Could you check a few things on this model? Use its own coordinates, in mm. A direction names the side the tool comes from. Round coordinates to 2 decimals unless told otherwise and drop trailing zeros. Order: outer loops, then holes, each group sorted by start corner. A loop starts at its lowest first (then second) coordinate and runs counter-clockwise, first axis right, second up. Notation, with made-up numbers: (41.25, -37.5) - (89.25, -37.5) arc R24 cw to (89.25, -18.5) - close; hole circle Ø5 at (56, 68). An arc over 180 degrees is marked (long way). Return JSON: item names as keys, results as strings. Group by question number.
from build123d import *

# Parameters (mm, degrees)
SKETCH1_R           = 0.95
SKETCH1_R_2         = 2.5
SKETCH1_R_3         = 1.449999999
SKETCH1_R_4         = 1.45
SKETCH1_W           = 6.2
SKETCH1_H           = 3.4
BOSS_EXTRUDE1_DEPTH = 5.85
FILLET1_R           = 4


with BuildPart() as part:
    # Sketch1 → Boss-Extrude1 (new body)
    with BuildSketch(Plane.XY):
        with BuildLine():
            Line((576.616706289, 434.650231372), (532.426650002, 446.716128422))
            ThreePointArc((532.426650002, 446.716128422), (529.426650002, 450.550186325), (532.426650002, 454.384244227))
            Line((532.426650002, 454.384244227), (576.616706289, 466.450141278))
            ThreePointArc((576.616706289, 466.450141278), (587.144059076, 475.326320371), (587.176754813, 489.096238418))
            Line((587.176754813, 489.096238418), (568.014947547, 530.703594601))
            ThreePointArc((568.014947547, 530.703594601), (569.023643468, 535.466212845), (573.889065048, 535.63256443))
            Line((573.889065048, 535.63256443), (611.536899087, 509.536826494))
            ThreePointArc((611.536899087, 509.536826494), (640.276650002, 500.550186325), (669.016400917, 509.536826494))
            Line((669.016400917, 509.536826494), (706.664234956, 535.63256443))
            ThreePointArc((706.664234956, 535.63256443), (711.529656536, 535.466212845), (712.538352458, 530.703594601))
            Line((712.538352458, 530.703594601), (693.376545192, 489.096238418))
            ThreePointArc((693.376545192, 489.096238418), (693.409240928, 475.326320371), (703.936593716, 466.450141278))
            Line((703.936593716, 466.450141278), (748.126650002, 454.384244227))
            ThreePointArc((748.126650002, 454.384244227), (751.126650002, 450.550186325), (748.126650002, 446.716128422))
            Line((748.126650002, 446.716128422), (703.936593716, 434.650231372))
            ThreePointArc((703.936593716, 434.650231372), (693.409240928, 425.774052279), (693.376545192, 412.004134232))
            Line((693.376545192, 412.004134232), (712.538352458, 370.396778049))
            ThreePointArc((712.538352458, 370.396778049), (711.529656536, 365.634159805), (706.664234956, 365.46780822))
            Line((706.664234956, 365.46780822), (683.276650002, 381.679000803))
            ThreePointArc((683.276650002, 381.679000803), (677.397639803, 388.334757147), (675.276650002, 396.958170375))
            Line((675.276650002, 396.958170375), (675.276650002, 489.550186325))
            Line((675.276650002, 489.550186325), (605.276650002, 489.550186325))
            Line((605.276650002, 489.550186325), (605.276650002, 396.958170375))
            ThreePointArc((605.276650002, 396.958170375), (603.155660202, 388.334757147), (597.276650002, 381.679000803))
            Line((597.276650002, 381.679000803), (573.889065048, 365.46780822))
            ThreePointArc((573.889065048, 365.46780822), (569.023643468, 365.634159805), (568.014947547, 370.396778049))
            Line((568.014947547, 370.396778049), (587.176754813, 412.004134232))
            ThreePointArc((587.176754813, 412.004134232), (587.144059076, 425.774052279), (576.616706289, 434.650231372))
        make_face()
        with Locations((533.376650002, 450.550186325)):
            Circle(SKETCH1_R, mode=Mode.SUBTRACT)
        with Locations((575.997889034, 527.154630637)):
            Circle(SKETCH1_R_2, mode=Mode.SUBTRACT)
        with Locations((547.176650002, 450.550186325)):
            Circle(SKETCH1_R, mode=Mode.SUBTRACT)
        with Locations((540.276650002, 450.550186325)):
            Circle(SKETCH1_R_2, mode=Mode.SUBTRACT)
        with Locations((590.276650002, 460.550186325)):
            Circle(SKETCH1_R_3, mode=Mode.SUBTRACT)
        with Locations((571.562654527, 532.440337294)):
            Circle(SKETCH1_R, mode=Mode.SUBTRACT)
        with Locations((580.43312354, 521.868923979)):
            Circle(SKETCH1_R, mode=Mode.SUBTRACT)
        with Locations(Location((682.276650002, 470.550186325, 0), (0, 0, 180))):
            Circle(SKETCH1_R_4, mode=Mode.SUBTRACT)
        with Locations((630.276650002, 494.550186325)):
            Circle(SKETCH1_R_4, mode=Mode.SUBTRACT)
        with Locations((620.276650002, 494.550186325)):
            Circle(SKETCH1_R_4, mode=Mode.SUBTRACT)
        with Locations((580.43312354, 379.231448671)):
            Circle(SKETCH1_R, mode=Mode.SUBTRACT)
        with Locations((575.997889034, 373.945742013)):
            Circle(SKETCH1_R_2, mode=Mode.SUBTRACT)
        with Locations((571.562654527, 368.660035356)):
            Circle(SKETCH1_R, mode=Mode.SUBTRACT)
        with Locations(Location((590.276650002, 430.550186325, 0), (0, 0, 180))):
            Circle(SKETCH1_R_3, mode=Mode.SUBTRACT)
        with Locations(Location((590.276650002, 440.550186325, 0), (0, 0, 180))):
            Circle(SKETCH1_R_3, mode=Mode.SUBTRACT)
        with Locations((590.276650002, 470.550186325)):
            Circle(SKETCH1_R_3, mode=Mode.SUBTRACT)
        with Locations(Location((682.276650002, 430.550186325, 0), (0, 0, 180))):
            Circle(SKETCH1_R_4, mode=Mode.SUBTRACT)
        with Locations(Location((708.990645478, 368.660035356, 0), (0, 0, 180))):
            Circle(SKETCH1_R, mode=Mode.SUBTRACT)
        with Locations(Location((704.555410971, 373.945742013, 0), (0, 0, 180))):
            Circle(SKETCH1_R_2, mode=Mode.SUBTRACT)
        with Locations(Location((700.120176464, 379.231448671, 0), (0, 0, 180))):
            Circle(SKETCH1_R, mode=Mode.SUBTRACT)
        with Locations(Location((660.276650002, 494.550186325, 0), (0, 0, 180))):
            Circle(SKETCH1_R_4, mode=Mode.SUBTRACT)
        with Locations(Location((650.276650002, 494.550186325, 0), (0, 0, 180))):
            Circle(SKETCH1_R_4, mode=Mode.SUBTRACT)
        with Locations(Location((700.120176464, 521.868923979, 0), (0, 0, 180))):
            Circle(SKETCH1_R, mode=Mode.SUBTRACT)
        with Locations(Location((708.990645478, 532.440337294, 0), (0, 0, 180))):
            Circle(SKETCH1_R, mode=Mode.SUBTRACT)
        with Locations(Location((690.276650002, 450.550186325, 0), (0, 0, 180))):
            Circle(SKETCH1_R_3, mode=Mode.SUBTRACT)
        with Locations(Location((740.276650002, 450.550186325, 0), (0, 0, 180))):
            Circle(SKETCH1_R_2, mode=Mode.SUBTRACT)
        with Locations(Location((733.376650002, 450.550186325, 0), (0, 0, 180))):
            Circle(SKETCH1_R, mode=Mode.SUBTRACT)
        with Locations(Location((704.555410971, 527.154630637, 0), (0, 0, 180))):
            Circle(SKETCH1_R_2, mode=Mode.SUBTRACT)
        with Locations(Location((747.176650002, 450.550186325, 0), (0, 0, 180))):
            Circle(SKETCH1_R, mode=Mode.SUBTRACT)
        with Locations(Location((690.276650002, 470.550186325, 0), (0, 0, 180))):
            Circle(SKETCH1_R_3, mode=Mode.SUBTRACT)
        with Locations((640.276650002, 494.550186325)):
            Circle(SKETCH1_R_4, mode=Mode.SUBTRACT)
        with Locations((690.276650002, 440.550186325)):
            Circle(SKETCH1_R_3, mode=Mode.SUBTRACT)
        with Locations((690.276650002, 430.550186325)):
            Circle(SKETCH1_R_3, mode=Mode.SUBTRACT)
        with Locations(Location((690.276650002, 460.550186325, 0), (0, 0, 180))):
            Circle(SKETCH1_R_3, mode=Mode.SUBTRACT)
        with Locations((590.276650002, 450.550186325)):
            Circle(SKETCH1_R_3, mode=Mode.SUBTRACT)
        with Locations((598.276650002, 430.550186325)):
            Circle(SKETCH1_R_4, mode=Mode.SUBTRACT)
        with Locations((598.276650002, 470.550186325)):
            Circle(SKETCH1_R_4, mode=Mode.SUBTRACT)
        with BuildLine():
            Line((549.378217697, 453.82975942), (576.389421361, 461.205047663))
            ThreePointArc((576.389421361, 461.205047663), (580.337323048, 460.434368256), (582.12067631, 456.828882764))
            Line((582.12067631, 456.828882764), (582.12067631, 444.271489885))
            ThreePointArc((582.12067631, 444.271489885), (580.337323048, 440.666004394), (576.389421361, 439.895324987))
            Line((576.389421361, 439.895324987), (549.378217697, 447.27061323))
            ThreePointArc((549.378217697, 447.27061323), (551.126650002, 450.550186325), (549.378217697, 453.82975942))
        make_face(mode=Mode.SUBTRACT)
        with BuildLine():
            Line((590.015887334, 402.739634304), (597.776650002, 402.739634304))
            ThreePointArc((597.776650002, 402.739634304), (599.544416955, 402.007401257), (600.276650002, 400.239634304))
            Line((600.276650002, 400.239634304), (600.276650002, 396.958170375))
            ThreePointArc((600.276650002, 396.958170375), (598.726100476, 390.65402441), (594.428250258, 385.788333948))
            Line((594.428250258, 385.788333948), (586.310038369, 380.161164806))
            ThreePointArc((586.310038369, 380.161164806), (584.257709818, 383.789413107), (580.328199648, 385.180523471))
            Line((580.328199648, 385.180523471), (587.745126051, 401.285408274))
            ThreePointArc((587.745126051, 401.285408274), (588.667635675, 402.34491753), (590.015887334, 402.739634304))
        make_face(mode=Mode.SUBTRACT)
        with Locations((598.276650002, 420.515790438)):
            Rectangle(SKETCH1_W, SKETCH1_H, mode=Mode.SUBTRACT)
        with BuildLine():
            Line((694.243261635, 380.161164806), (686.125049746, 385.788333948))
            ThreePointArc((686.125049746, 385.788333948), (681.827199528, 390.65402441), (680.276650002, 396.958170375))
            Line((680.276650002, 396.958170375), (680.276650002, 400.239634304))
            ThreePointArc((680.276650002, 400.239634304), (681.008883049, 402.007401257), (682.776650002, 402.739634304))
            Line((682.776650002, 402.739634304), (690.53741267, 402.739634304))
            ThreePointArc((690.53741267, 402.739634304), (691.88566433, 402.34491753), (692.808173953, 401.285408274))
            Line((692.808173953, 401.285408274), (700.225100356, 385.180523471))
            ThreePointArc((700.225100356, 385.180523471), (696.295590186, 383.789413107), (694.243261635, 380.161164806))
        make_face(mode=Mode.SUBTRACT)
        with BuildLine():
            Line((579.335965232, 518.07435633), (591.048633694, 492.641829961))
            ThreePointArc((591.048633694, 492.641829961), (594.150648115, 490.133983107), (598.026414137, 491.077501553))
            Line((598.026414137, 491.077501553), (607.701712221, 499.196040607))
            ThreePointArc((607.701712221, 499.196040607), (609.303916208, 502.849084775), (607.372828334, 506.339455663))
            Line((607.372828334, 506.339455663), (584.360562722, 522.29049423))
            ThreePointArc((584.360562722, 522.29049423), (582.972134599, 518.843048429), (579.335965232, 518.07435633))
        make_face(mode=Mode.SUBTRACT)
        with Locations((682.276650002, 480.550186325)):
            Rectangle(SKETCH1_W, SKETCH1_H, mode=Mode.SUBTRACT)
        with BuildLine():
            Line((672.851587783, 499.196040607), (682.526885868, 491.077501553))
            ThreePointArc((682.526885868, 491.077501553), (686.402651889, 490.133983107), (689.50466631, 492.641829961))
            Line((689.50466631, 492.641829961), (701.217334773, 518.07435633))
            ThreePointArc((701.217334773, 518.07435633), (697.581165406, 518.843048429), (696.192737283, 522.29049423))
            Line((696.192737283, 522.29049423), (673.18047167, 506.339455663))
            ThreePointArc((673.18047167, 506.339455663), (671.249383797, 502.849084775), (672.851587783, 499.196040607))
        make_face(mode=Mode.SUBTRACT)
        with BuildLine():
            Line((698.432623695, 456.828882764), (698.432623695, 444.271489885))
            ThreePointArc((698.432623695, 444.271489885), (700.215976956, 440.666004394), (704.163878644, 439.895324987))
            Line((704.163878644, 439.895324987), (731.175082307, 447.27061323))
            ThreePointArc((731.175082307, 447.27061323), (729.426650002, 450.550186325), (731.175082307, 453.82975942))
            Line((731.175082307, 453.82975942), (704.163878644, 461.205047663))
            ThreePointArc((704.163878644, 461.205047663), (700.215976956, 460.434368256), (698.432623695, 456.828882764))
        make_face(mode=Mode.SUBTRACT)
        with Locations((682.276650002, 420.515790438)):
            Rectangle(SKETCH1_W, SKETCH1_H, mode=Mode.SUBTRACT)
        with Locations((598.276650002, 480.550186325)):
            Rectangle(SKETCH1_W, SKETCH1_H, mode=Mode.SUBTRACT)
    extrude(amount=BOSS_EXTRUDE1_DEPTH)

    # Fillet1
    fillet1_edges = [part.edges().sort_by_distance(p)[0] for p in [
        (675.276650002, 489.550186325, 2.925),
        (605.276650002, 489.550186325, 2.925),
    ]]
    fillet(fillet1_edges, radius=FILLET1_R)


solid = part.part
1) I want a section at B-B, the plane z = 4. Give the number of separate pieces and of enclosed holes in the cut face, plus the area to 3 significant figures.
2) I want a section at C-C, the plane x = 626.5. List the corners of the cut face in (y, z) for me.
3) If I drill on line 1 along X through (y, z) = (396, 2.8); line 2 along X through (y, z) = (512.5, 4.7); line 3 along Y through (x, z) = (600.5, 4.1), over which ranges is the centre line in solid material (lowest first)? Write a range as from..to.
4) We'd pull the mould along X, two halves only. Please class faces 3 (the flat face through (554.83, 440.6, 2.88)), 4 (the flat face through (598, 418.816, 3)): +X half, -X half, draft (parallel to the pull), parting line (faces both ways), or undercut.
5) I want a section at A-A, the plane y = 425. List the corners of the cut face in (x, z) for me.
6) Will these pins go through, and if not, where does the flat tip stop? pin 1 (2 mm diameter, centred on x = 682, y = 494, fed in from -Z); pin 2 (1.8 mm diameter, centred on x = 598, z = 4, fed in from +Y); pin 3 (1 mm diameter, centred on y = 409.5, z = 5.5, fed in from -X); pin 4 (2 mm diameter, centred on x = 577, z = 5, fed in from -Y).
7) For faces 1 (the flat face through (641, 489.55, 3)), 2 (the cylindrical face through (580.38, 440.7, 2.88)), which set-ups out of +Z, -Z, +X, -X, +Y, -Y let a thin tool reach every point of the face, with its end or its side?
Outcome:
{
 "1": {"separate pieces": "1", "enclosed holes": "47", "area": "7,500 mm^2"},
 "2": {"outline": "(489.55, 0) - (502.47, 0) - (502.47, 5.85) - (489.55, 5.85) - close"},
 "3": {"line 1": "579.81..585.31, 600.24..605.25, 675.3..680.31, 695.24..700.75", "line 2": "576.4..581.9, 598.49..607.26, 673.29..682.07, 698.65..704.15", "line 3": "384.52..418.82, 422.22..478.85, 482.25..493.15, 511.1..517.19"},
 "4": {"face 3": "-X half", "face 4": "undercut"},
 "5": {"outline": "(587.48, 0) - (605.28, 0) - (605.28, 5.85) - (587.48, 5.85) - close; (675.28, 0) - (693.07, 0) - (693.07, 5.85) - (675.28, 5.85) - close"},
 "6": {"pin 1": "through", "pin 2": "y = 519.54", "pin 3": "x = 585.79", "pin 4": "y = 366.93"},
 "7": {"face 1": "+Z, -Z, -Y", "face 2": "+Z, -Z"}
}
